Can you work these out from the model? Positions are in its coordinate system, mm. Face numbers are marked on the shaded views. A direction names the side the tool comes from. Coordinates: 2 decimals unless noted, no trailing zeros. Write each loop counter-clockwise with the first axis right and the second up, starting at its lowest first coordinate (ties: lowest second). Pieces come first, ordered by that corner, then holes.
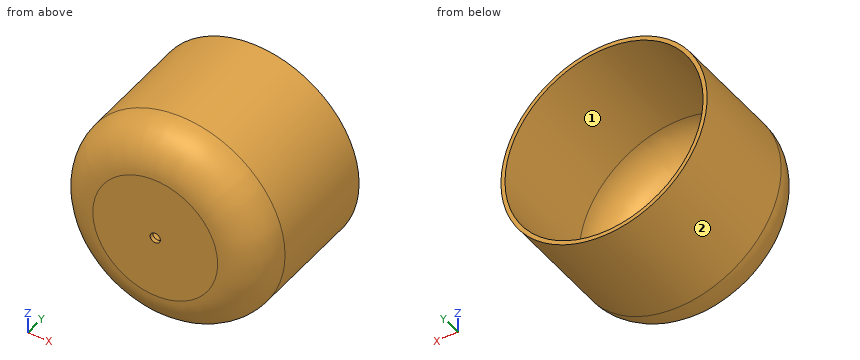
```python
from build123d import *

# Parameters (mm, degrees)
F0_R     = 64.391554
F1_DEPTH = 95.8381
F2_R     = 25.4
F3_T     = -2.54
F5_D     = 6.35


with BuildPart() as f1:
    # F0 (on Front) → F1 (new body)
    with BuildSketch(Plane.XZ):
        Circle(F0_R)
    extrude(amount=F1_DEPTH)

    # F2
    f2_edges = [f1.edges().sort_by_distance(p)[0] for p in [
        (-64.391554, -95.8381, 0),
    ]]
    fillet(f2_edges, radius=F2_R)

    # F3
    f3_openings = [f1.faces().sort_by_distance(p)[0] for p in [
        (0, 0, 0),
    ]]
    offset(amount=F3_T, openings=f3_openings)

    # F5 (through all)
    with Locations(Plane.XZ.offset(95.8381)):
        with Locations((0, 0)):
            Hole(F5_D / 2)


solid = f1.part
```
1. I'm going to push flat-ended pins straight in: P1, Ø1, axis at x = 3.5, y = -17.5, coming from the -Z side; P2, Ø5.5, axis at x = 0, z = 0, coming from the +Y side; P3, Ø12, axis at x = 35, z = -40, coming from the +Y side; P4, Ø2, axis at x = -27, y = -24, coming from the -Z side. Where does each tip first touch, or does it pass through?
2. If we section it at C-C, the plane y = -38.5: List the corners of the cut face in (x, z) for me, plus the area to 3 significant figures.
3. If we section it at A-A, the plane x = 0: List the corners of the cut face in (y, z) for me (3 decimals), plus the area to 3 significant figures.
4. If we section it at B-B, the plane z = 0: List the corners of the cut face in (x, y) for me (3 decimals).
5. If I drill on L1, parallel to Z at x = -0.5, y = -21; L2, parallel to X at y = -10.5, z = 19.5; L3, parallel to Z at x = -11, y = -55, over which ranges is the centre line in solid material (lowest first)?
6. If we section it at D-D, the plane y = -88: List the corners of the cut face in (x, z) for me.
7. Which directions (+Z, -Z, +X, -X, +Y, -Y) give clear straight access to the entire face, cutting with the end or side of a thin tool? Please do the marked faces 1 and 2.
Answers:
1. P1: stops at z = -64.32
1. P2: passes through
1. P3: stops at y = -81.22
1. P4: stops at z = -58.91
2. outline: circle Ø128.78 at (0, 0); hole circle Ø123.7 at (0, 0)
2. area: 1,010 mm2
3. outline: (-95.838, -38.992) arc R25.4 ccw to (-70.438, -64.392) - (0, -64.392) - (0, -61.852) - (-70.438, -61.852) arc R22.86 cw to (-93.298, -38.992) - (-93.298, -3.175) - (-95.838, -3.175) - close; (-95.838, 3.175) - (-93.298, 3.175) - (-93.298, 38.992) arc R22.86 cw to (-70.438, 61.852) - (0, 61.852) - (0, 64.392) - (-70.438, 64.392) arc R25.4 ccw to (-95.838, 38.992) - close
3. area: 732 mm2
4. outline: (-64.392, -70.438) arc R25.4 ccw to (-38.992, -95.838) - (-3.175, -95.838) - (-3.175, -93.298) - (-38.992, -93.298) arc R22.86 cw to (-61.852, -70.438) - (-61.852, 0) - (-64.392, 0) - close; (3.175, -95.838) - (38.992, -95.838) arc R25.4 ccw to (64.392, -70.438) - (64.392, 0) - (61.852, 0) - (61.852, -70.438) arc R22.86 cw to (38.992, -93.298) - (3.175, -93.298) - close
5. L1: z = -64.39 to -61.85, 61.85 to 64.39
5. L2: x = -61.37 to -58.7, 58.7 to 61.37
5. L3: z = -63.45 to -60.87, 60.87 to 63.45
6. outline: circle Ø114.68 at (0, 0); hole circle Ø107.25 at (0, 0)
7. face 1: +Y
7. face 2: +Y, -Y
